from build123d import *

# Parameters (mm, degrees)
EXTRUDE1_REACH           = 62.064
SKETCH11_W               = 7
SKETCH11_H               = 0.833333333
POINT_CUT_EXTRUDE8_DEPTH = 53.158412553


with BuildPart() as part:
    # Sketch1 → base-Revolve (revolve)
    with BuildSketch(Plane.XY, mode=Mode.PRIVATE) as base_revolve_sk:
        with BuildLine():
            Line((0, 10.5), (-1.2, 10.5))
            Line((-1.2, 10.5), (-2.499678785, 6.5))
            Line((-2.499678785, 6.5), (-8.2, 6.5))
            Line((-8.2, 6.5), (-8.2, 0))
            Line((-8.2, 0), (-6.8, 0))
            Line((-6.8, 0), (0, 0))
            Line((0, 0), (50, 0))
            Line((50, 0), (50, 5))
            Line((50, 5), (3, 5))
            Line((3, 5), (2, 4))
            Line((2, 4), (0.4, 4))
            ThreePointArc((0.4, 4), (0.117157288, 4.117157288), (0, 4.4))
            Line((0, 4.4), (0, 10.5))
        make_face()
    revolve(base_revolve_sk.sketch.rotate(Axis((0, 0, 0), (1, 0, 0)), 90), axis=Axis((0, 0, 0), (1, 0, 0)))

    # Extrude1: up to this cone (the profile starts outside it)
    extrude1_end = Plane(origin=(-8.2, 0, 0), z_dir=(1, 0, 0)).offset(3.58834419) * Cone(3.078e-06, 181.50840806, 58.97565581, align=(Align.CENTER, Align.CENTER, Align.MIN), mode=Mode.PRIVATE)
    # Sketch15 → Extrude1 (add, up to the surface)
    with BuildSketch(Plane.ZY.offset(8.2), mode=Mode.PRIVATE) as extrude1_sk1:
        Polygon((-3.75277675, 6.5), (-7.505553499, 0), (-3.75277675, -6.5), (3.75277675, -6.5), (7.505553499, 0), (3.75277675, 6.5), align=None)
    extrude1_tool1 = extrude(extrude1_sk1.sketch, amount=-EXTRUDE1_REACH, mode=Mode.PRIVATE) - extrude1_end
    add(extrude1_tool1.solids().sort_by_distance((-8.2, 0, 0))[0])

    # Sketch8 → point_Cut-Revolve1 (revolve, cut)
    with BuildSketch(Plane.XY, mode=Mode.PRIVATE) as point_cut_revolve1_sk:
        Polygon((50, 0), (50.508, 0), (50.508, 5.508), (48.337231225, 5.508), (48.337231225, 5), (50, 4.04), align=None)
    revolve(point_cut_revolve1_sk.sketch.rotate(Axis((0, 0, 0), (1, 0, 0)), 90), axis=Axis((0, 0, 0), (1, 0, 0)), mode=Mode.SUBTRACT)

    # Sketch11 → point_Cut-Extrude8 (cut, through all)
    with BuildSketch(Plane.XY):
        with Locations((46.5, -0.416666667)):
            Rectangle(SKETCH11_W, SKETCH11_H)
    extrude(amount=POINT_CUT_EXTRUDE8_DEPTH, mode=Mode.SUBTRACT)


solid = part.part
Build history of the part. All positions in model axes, mm. A direction names the side the tool comes from. Give positions to 0.01 mm unless a question says otherwise; leave off trailing zeros. Loops run counter-clockwise (first coordinate to the right, second up) from the corner with the lowest first, then second, coordinate; pieces in that order, holes last. Notation, with made-up numbers: (-29.75, 87.25) - (6.25, 87.25) arc R22 cw to (6.25, 98.25) - close; hole circle Ø9 at (7, 47.5). An arc over 180 degrees is marked (long way). Write item = value, one per line. Start each with the question number.
1) Tool access for faces 5 (the flat face through (-5.2, -3.3, 5.6)), 6 (the cylindrical face through (25, 0, -5)), 7 (the cylindrical face through (1.189, 3.905, -0.867)), 8 (the flat face through (-5.23, 3.2, 5.66)), 9 (the flat face through (-5.23, -3.2, -5.66)): list every direction of +Z, -Z, +X, -X, +Y, -Y with a clear straight run to the whole face (end or side of a thin tool).
2) Drop flat-ended pins along their axis: pin 1 Ø3 at (x, y) = (41, 6) entering from +Z; pin 2 Ø2 at (y, z) = (5.5, -1.5) entering from +X; pin 3 Ø12 at (x, z) = (22.5, -7.5) entering from -Y. Give the stop position or say it passes through.
3) Probe probe 1 along X at (y, z) = (-4.25, -4); probe 2 along Y at (x, z) = (35, -2); probe 3 along Z at (x, y) = (5, 1.5). List the from-to ranges inside material, lowest first. Write a range as from..to.
4) Pull direction Y, two halves, no side cores. Call faces 1 (the flat face through (0, 0, -5)), 2 (the flat face through (46, 0, 2)), 3 (the flat face through (46, -0.833, 2)), 4 (the flat face through (-5.2, 3.3, -5.6)): +Y half, -Y half, draft (parallel to the pull), parting line (faces both ways), or undercut.
5) Band-saw the part on A-A on x = 38. Give the cut face in (y, z).
Final values:
q1.face_5 = +Z, -X, -Y
q1.face_6 = +X
q1.face_7 = none
q1.face_8 = +Z, -X, +Y
q1.face_9 = -Z, -X, -Y
q2.pin_1 = 2.18
q2.pin_2 = 48.86
q2.pin_3 = -4.77
q3.probe_1 = -8.2..0
q3.probe_2 = -4.58..4.58
q3.probe_3 = -4.77..4.77
q4.face_1 = draft
q4.face_2 = undercut
q4.face_3 = undercut
q4.face_4 = +Y half
q5.outline = circle Ø10 at (0, 0)
